from build123d import *

# Parameters (mm, degrees)
SKETCH1_W           = 24
SKETCH1_H           = 90
BOSS_EXTRUDE1_DEPTH = 4
SKETCH2_R           = 4
SKETCH2_R_2         = 1.5
CUT_EXTRUDE1_DEPTH  = 4
FILLET1_R           = 4
SKETCH3_R           = 1.5
CUT_EXTRUDE2_DEPTH  = 4


with BuildPart() as part:
    # Sketch1 → Boss-Extrude1 (new body)
    with BuildSketch(Plane.XY):
        with Locations((-45.296675466, -10.049681021)):
            Rectangle(SKETCH1_W, SKETCH1_H)
    extrude(amount=BOSS_EXTRUDE1_DEPTH)

    # Sketch2 → Cut-Extrude1 (cut)
    with BuildSketch(Plane.XY.offset(4)):
        with Locations((-45.296675466, -43.049681021)):
            Circle(SKETCH2_R)
        with Locations((-37.296675466, -43.049681021)):
            Circle(SKETCH2_R_2)
        with Locations((-45.296675466, -51.049681021)):
            Circle(SKETCH2_R_2)
        with Locations((-53.296675466, -43.049681021)):
            Circle(SKETCH2_R_2)
        with Locations((-45.296675466, -35.049681021)):
            Circle(SKETCH2_R_2)
        with Locations((-45.296675466, 30.950318979)):
            Circle(SKETCH2_R_2)
        with Locations((-37.296675466, 22.950318979)):
            Circle(SKETCH2_R_2)
        with Locations((-45.296675466, 14.950318979)):
            Circle(SKETCH2_R_2)
        with Locations((-53.296675466, 22.950318979)):
            Circle(SKETCH2_R_2)
        with Locations((-45.296675466, 22.950318979)):
            Circle(SKETCH2_R)
    extrude(amount=-CUT_EXTRUDE1_DEPTH, mode=Mode.SUBTRACT)

    # Fillet1
    fillet1_edges = [part.edges().sort_by_distance(p)[0] for p in [
        (-57.296675466, 34.950318979, 2),
        (-57.296675466, -55.049681021, 2),
        (-33.296675466, -55.049681021, 2),
        (-33.296675466, 34.950318979, 2),
    ]]
    fillet(fillet1_edges, radius=FILLET1_R)

    # Sketch3 → Cut-Extrude2 (cut)
    with BuildSketch(Plane.XY.offset(4)):
        with Locations((-45.296675466, -5.049681021)):
            Circle(SKETCH3_R)
    extrude(amount=-CUT_EXTRUDE2_DEPTH, mode=Mode.SUBTRACT)


solid = part.part
Geometry: final body of the model. Coordinates: model frame, mm. Give positions to 0.01 mm unless a question says otherwise; leave off trailing zeros. Loops run counter-clockwise (first coordinate to the right, second up) from the corner with the lowest first, then second, coordinate; pieces in that order, holes last. Notation, with made-up numbers: (82, 87.5) - (119, 87.5) arc R20 cw to (119, 113.5) - close; hole circle Ø2 at (-1.75, -40). An arc over 180 degrees is marked (long way). One line per question, with ' | ' between items. Start each with the question number.
(1) Section query A-A on x = -45.75. Count the separate pieces of the cut face and the enclosed holes in it, then the cut area to 3 significant figures.
(2) Pull-direction query (X, two-part tool) for faces 1 (the cylindrical face through (-46.402, 31.964, 2.028)), 2 (the cylindrical face through (-34.5, 33.81, 2.03)), 3 (the flat face through (-57.297, -11, 2)); classes: released by +X, released by -X, zero draft, split by the parting line, or undercut.
(3) Ray query, line 1 (Y direction, x = -47.75, z = 0.7); line 2 (Y direction, x = -54.5, z = 1.3); line 3 (X direction, y = -42.5, z = 2.7). Return the intervals inside material, ascending. Write a range as from..to.
(4) Contact query for a flat-ended pin moving along its axis: pin 1 (2.5 mm diameter, centred on x = -45.3, y = 30.95, fed in from -Z). Output: stop coordinate, or through.
(5) Section query C-C on x = -34.75. Return loops of the section in (y, z).
The answers:
1) separate pieces: 8 | enclosed holes: 0 | area: 239 mm2
2) face 1: undercut | face 2: released by +X | face 3: released by -X
3) line 1: -55.05..-46.21, -39.89..19.79, 26.11..34.95 | line 2: -54.86..-43.95, -42.15..22.05, 23.85..34.77 | line 3: -57.3..-54.69, -51.9..-49.26, -41.33..-38.69, -35.9..-33.3
4) pin 1: through
5) outline: (-54.13, 0) - (34.03, 0) - (34.03, 4) - (-54.13, 4) - close
